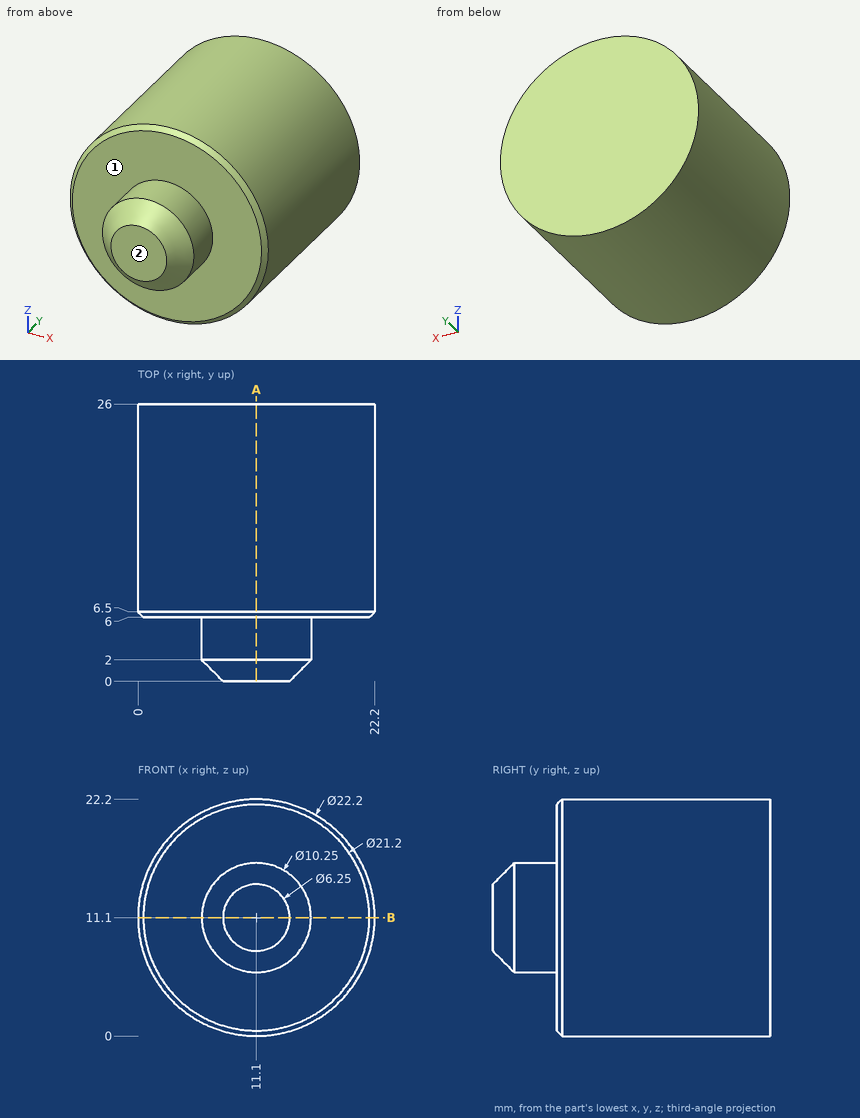
Part print with two shaded views. Sizes in mm from the minimum x, y, z corner. A direction names the side the tool comes from. Give positions to 0.01 mm unless a question says otherwise; leave off trailing zeros. Order: outer loops, then holes, each group sorted by start corner. A loop starts at its lowest first (then second) coordinate and runs counter-clockwise, first axis right, second up. Notation, with made-up numbers: M 12,-39.5 L 35,-39.5 A33 ccw 35,-3.5 Z; hole C -7.5,19.25 d6. An arc over 180 degrees is marked long. Write item = value, one per line.
Q1. Drill centre lines: line 1 (Y direction, x = 13.25, z = 5); line 2 (X direction, y = 6.5, z = 11.5); line 3 (X direction, y = 9, z = 3). Where is each one in solid material? Low to high. Write a range as [from, to].
Derived:
line_1 = [6, 26]
line_2 = [0.01, 22.19]
line_3 = [3.51, 18.69]
Q2. Tool access for the marked faces 1 and 2: list every direction of +Z, -Z, +X, -X, +Y, -Y with a clear straight run to the whole face (end or side of a thin tool).
Derived:
face_1 = -Y
face_2 = +Z, -Z, +X, -X, -Y
Q3. Flat gauge pins, fed straight in: pin 1 (1.5 mm diameter, centred on x = 16, y = 23, fed in from +Z) (3 decimals); pin 2 (10 mm diameter, centred on x = 5.5, z = 14.5, fed in from -Y); pin 3 (8 mm diameter, centred on x = 6, y = 13, fed in from -Z); pin 4 (4 mm diameter, centred on y = 22.5, z = 17, fed in from -X). Where does each tip first touch, or does it go through?
Derived:
pin_1 = 21.395
pin_2 = 0
pin_3 = 0.05
pin_4 = 0.71
Q4. Cut at B-B, the plane z = 11.1. List the corners of the cut face in (x, y) (3 decimals).
Derived:
outline = M 0,6.5 L 0.5,6 L 5.975,6 L 5.975,2 L 7.975,0 L 14.225,0 L 16.225,2 L 16.225,6 L 21.7,6 L 22.2,6.5 L 22.2,26 L 0,26 Z
Q5. Cut at A-A, the plane x = 11.1. List the corners of the cut face in (y, z) (3 decimals).
Derived:
outline = M 0,7.975 L 2,5.975 L 6,5.975 L 6,0.5 L 6.5,0 L 26,0 L 26,22.2 L 6.5,22.2 L 6,21.7 L 6,16.225 L 2,16.225 L 0,14.225 Z
